Design review of the part shown in the three views and the two pictorial views. Dimensions are in mm from the part's minimum x, y and z. A direction names the side the tool comes from. Round coordinates to 2 decimals unless told otherwise and drop trailing zeros. Loops run counter-clockwise (first coordinate to the right, second up) from the corner with the lowest first, then second, coordinate; pieces in that order, holes last. Notation, with made-up numbers: M 20,63 L 57,63 A14 cw 57,77 Z; hole C 46.5,-20 d10. An arc over 180 degrees is marked long. One line per question, with ' | ' between items. Start each with the question number.
1) We need section C-C (y = 36.5). Give the boundary of the cut face in (x, z), and give its area (3 significant figures).
2) Mouldability with a two-part tool opening along Y and no side actions: class the marked faces 1, 2 and 3 as pulls with the +Y half, pulls with the -Y half, needs draft (parallel to the pull), parting line crosses it, or undercut.
3) We need section B-B (z = 2.2). Give the boundary of the cut face in (x, y).
4) For probe 1 along Y at (x, z) = (15.5, 2.9); probe 2 along X at (y, z) = (22, 0.5); probe 3 along X at (y, z) = (15.5, 2.8), list the stretches that pass through material, from the lowest coordinate up. Write a range as from..to.
5) We need section A-A (x = 15.5). Give the boundary of the cut face in (y, z).
6) For the marked faces 4, 5, 6 and 7, list the 3-axis set-ups (+Z, -Z, +X, -X, +Y, -Y) from which the entire face can be reached by the end or side of a thin tool; tool diameter is ignored.
7) For pin 1 Ø0.9 at (y, z) = (1.5, 3) entering from +X; pin 2 Ø1 at (y, z) = (27.5, 0.5) entering from +X; pin 3 Ø1.2 at (y, z) = (21, 2) entering from -X, all flat-tipped, find the tip position at first contact; note any pin that passes through.
8) We need section D-D (x = 21.5). Give the boundary of the cut face in (y, z), and give its area (3 significant figures).
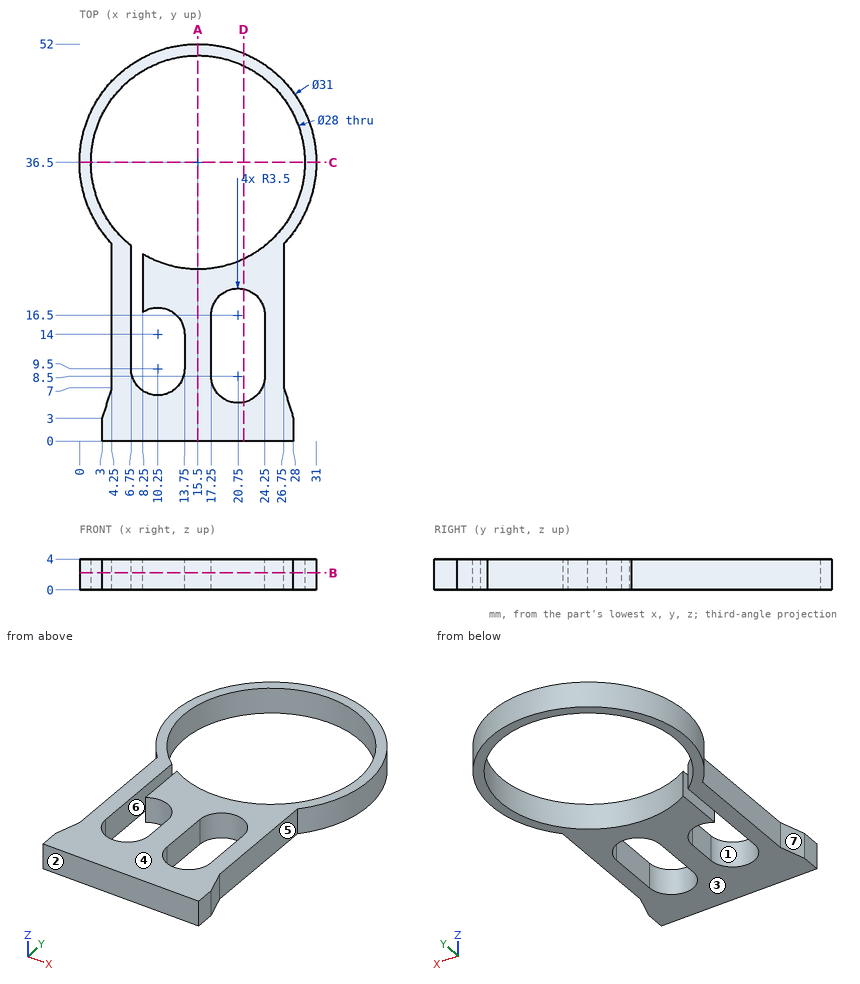
Answers below:
1) outline: M 0,0 L 1.5,0 L 1.5,4 L 0,4 Z; M 29.5,0 L 31,0 L 31,4 L 29.5,4 Z | area: 12.0 mm^2
2) face 1: undercut | face 2: pulls with the -Y half | face 3: needs draft
3) outline: M 3,0 L 28,0 L 28,3 L 26.75,7 L 26.75,25.84 A15.5 ccw long 4.25,25.84 L 4.25,7 L 3,3 Z; hole M 6.75,9.5 A3.5 ccw 13.75,9.5 L 13.75,14 A3.5 ccw 8.25,16.87 L 8.25,24.52 A14 ccw long 6.75,25.57 Z; hole M 17.25,8.5 A3.5 ccw 24.25,8.5 L 24.25,16.5 A3.5 ccw 17.25,16.5 Z
4) probe 1: 0..22.5, 50.5..52 | probe 2: 4.25..6.75, 8.25..26.75 | probe 3: 4.25..6.75, 13.41..17.25, 24.25..26.75
5) outline: M 0,0 L 22.5,0 L 22.5,4 L 0,4 Z; M 50.5,0 L 52,0 L 52,4 L 50.5,4 Z
6) face 4: +Z, +X, -X, +Y, -Y | face 5: +Z, -Z, +X | face 6: +Z, -Z | face 7: +Z, -Z, -X
7) pin 1: x = 28 | pin 2: x = 28.46 | pin 3: x = 4.25
8) outline: M 0,0 L 5.08,0 L 5.08,4 L 0,4 Z; M 19.92,0 L 23.85,0 L 23.85,4 L 19.92,4 Z; M 49.15,0 L 50.79,0 L 50.79,4 L 49.15,4 Z | area: 42.6 mm^2
